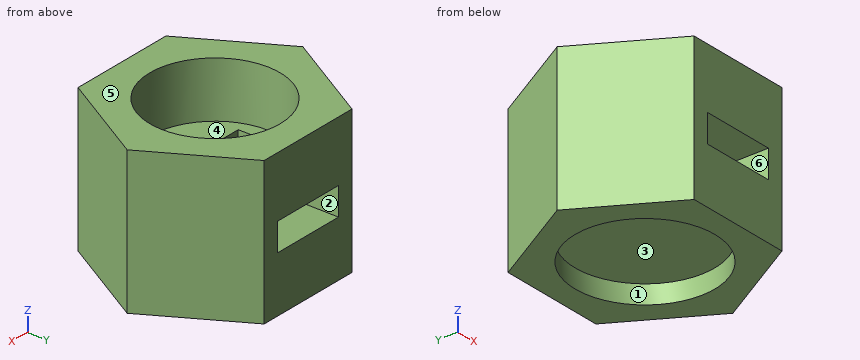
```python
from build123d import *

# Parameters (mm, degrees)
F1_DEPTH = 12.065
F2_W     = 10.16
F2_H     = 3.81
F3_DEPTH = 25.4010101543
F5_W     = 13.97
F5_H     = 5.08
F6_DEPTH = 8.255
F4_R     = 8.89
F7_DEPTH = 7.62
F8_R     = 9.525
F9_DEPTH = 2.54


# Not quite as in the source:
# - a feature names something its author has since deleted; it is built from what else it names


with BuildPart() as f1:
    # F0 (on Top) → F1 (new body)
    with BuildSketch(Plane.XY):
        Polygon((7.33235135, -12.7000050771), (14.6647027, 0), (7.33235135, 12.7000050771), (-7.33235135, 12.7000050771), (-14.6647027, 0), (-7.33235135, -12.7000050771), align=None)
    extrude(amount=F1_DEPTH)

    # F2 (on face) → F3 (cut, through all)
    with BuildSketch(Plane.XZ.offset(12.7000050771)):
        with Locations((0, 9.525)):
            Rectangle(F2_W, F2_H)
    extrude(amount=-F3_DEPTH, mode=Mode.SUBTRACT)

    # F5 (on face) → F6 (cut)
    with BuildSketch(Plane.XY.offset(12.065)):
        Rectangle(F5_W, F5_H)
    extrude(amount=-F6_DEPTH, mode=Mode.SUBTRACT)

    # F4 (on face) → F7 (join)
    with BuildSketch(Plane.XY.offset(12.065)):
        Polygon((-7.33235135, -12.7000050771), (7.33235135, -12.7000050771), (14.6647027, 0), (7.33235135, 12.7000050771), (-7.33235135, 12.7000050771), (-14.6647027, 0), align=None)
        Circle(F4_R, mode=Mode.SUBTRACT)
    extrude(amount=F7_DEPTH)

    # F8 (on face) → F9 (cut)
    with BuildSketch(Plane(origin=(0, 0, 0), x_dir=(1, 0, 0), z_dir=(0, 0, -1))):
        Circle(F8_R)
    extrude(amount=-F9_DEPTH, mode=Mode.SUBTRACT)


solid = f1.part
```
Input: part model. Units: mm. Frame: model coordinates. Face numbers are marked on the shaded views. A direction names the side the tool comes from. Give positions to 0.01 mm unless a question says otherwise; leave off trailing zeros. Order: outer loops, then holes, each group sorted by start corner. A loop starts at its lowest first (then second) coordinate and runs counter-clockwise, first axis right, second up. Notation, with made-up numbers: M 48.25,44 L 104.25,44 A12 ccw 104.25,59 Z; hole C -17.5,31 d1. An arc over 180 degrees is marked long. Return JSON: item names as keys, results as strings.
Item 1: First-contact query: P1, Ø5.5, axis at x = 0.5, y = -0.5, coming from the +Z side (3 decimals); P2, Ø9.5, axis at x = 4.5, y = 2, coming from the -Z side; P3, Ø3, axis at y = -6.5, z = 10.5, coming from the +X side; P4, Ø6, axis at x = 0, y = -4.5, coming from the -Z side. Flat tips, straight axial feed; report the tip coordinate or a pass-through.
Solutions:
{"P1": "z = 12.065", "P2": "z = 0", "P3": "x = 11.78", "P4": "z = 2.54"}
Item 2: Cut plane A-A (z = 9). Return loops of the section in (x, y) (3 decimals).
Solutions:
{"outline": "M -14.665,0 L -7.332,-12.7 L -5.08,-12.7 L -5.08,-2.54 L -6.985,-2.54 L -6.985,2.54 L -5.08,2.54 L -5.08,12.7 L -7.332,12.7 Z; M 5.08,-12.7 L 7.332,-12.7 L 14.665,0 L 7.332,12.7 L 5.08,12.7 L 5.08,2.54 L 6.985,2.54 L 6.985,-2.54 L 5.08,-2.54 Z"}
Item 3: Ray query, probe 1 along Y at (x, z) = (-6.5, 12); probe 2 along Y at (x, z) = (0, 0.65) (3 decimals); probe 3 along Z at (x, y) = (0.5, 5.75) (3 decimals). Return the intervals inside material, ascending.
Solutions:
{"probe 1": "-12.7 to -2.54, 2.54 to 12.7", "probe 2": "-12.7 to -9.525, 9.525 to 12.7", "probe 3": "2.54 to 7.62, 11.43 to 12.065"}
Item 4: Cut plane C-C (z = 13). Return loops of the section in (x, y), then the cut area to 3 significant figures.
Solutions:
{"outline": "M -14.66,0 L -7.33,-12.7 L 7.33,-12.7 L 14.66,0 L 7.33,12.7 L -7.33,12.7 Z; hole C 0,0 d17.78", "area": "310 mm^2"}
Item 5: Cut plane B-B (x = 0). Return loops of the section in (y, z) (3 decimals).
Solutions:
{"outline": "M -12.7,0 L -9.525,0 L -9.525,2.54 L 9.525,2.54 L 9.525,0 L 12.7,0 L 12.7,7.62 L 2.54,7.62 L 2.54,3.81 L -2.54,3.81 L -2.54,7.62 L -12.7,7.62 Z; M -12.7,11.43 L -2.54,11.43 L -2.54,12.065 L -8.89,12.065 L -8.89,19.685 L -12.7,19.685 Z; M 2.54,11.43 L 12.7,11.43 L 12.7,19.685 L 8.89,19.685 L 8.89,12.065 L 2.54,12.065 Z"}
Item 6: Cut plane D-D (y = -3.75). Return loops of the section in (x, z) (3 decimals).
Solutions:
{"outline": "M -12.5,0 L -8.756,0 L -8.756,2.54 L 8.756,2.54 L 8.756,0 L 12.5,0 L 12.5,19.685 L 8.06,19.685 L 8.06,12.065 L -8.06,12.065 L -8.06,19.685 L -12.5,19.685 Z; hole M -5.08,7.62 L 5.08,7.62 L 5.08,11.43 L -5.08,11.43 Z"}
Item 7: Pull-direction query (Z, two-part tool) for the marked faces 1, 2 and 3; classes: +Z half, -Z half, draft (parallel to the pull), parting line (faces both ways), or undercut.
Solutions:
{"face 1": "draft", "face 2": "undercut", "face 3": "-Z half"}
Item 8: Access query for the marked faces 4, 5 and 6. Directions: +Z, -Z, +X, -X, +Y, -Y. A direction counts if a zero-diameter tool reaches every point of the face in a straight line with its end or side. Return the directions, or none.
Solutions:
{"face 4": "+Z", "face 5": "+Z, +X, -X, +Y, -Y", "face 6": "+Y, -Y"}
